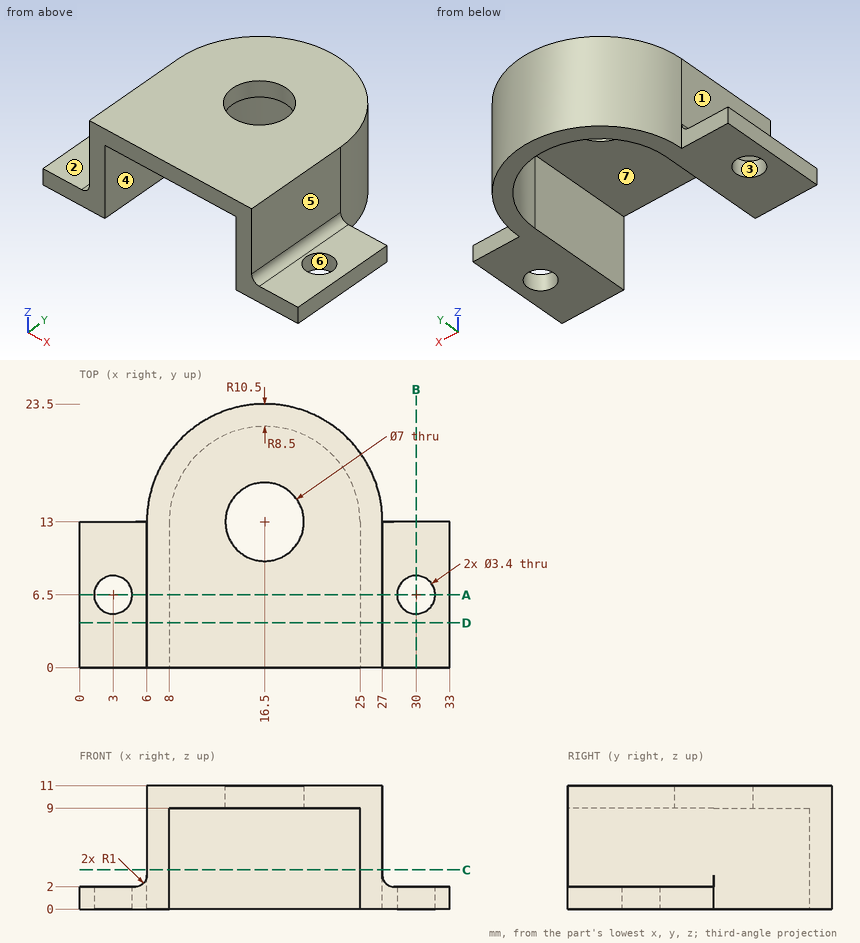
Could you check a few things on this drawing? It's one solid part, dimensions in mm from its lowest x, y, z. A direction names the side the tool comes from. Coordinates: 2 decimals unless noted, no trailing zeros. Order: outer loops, then holes, each group sorted by start corner. A loop starts at its lowest first (then second) coordinate and runs counter-clockwise, first axis right, second up.
1. If we section it at B-B (x = 30): Please give me the cut outline in (y, z).
2. For the marked faces 5, 6 and 7, which set-ups out of +Z, -Z, +X, -X, +Y, -Y let a thin tool reach every point of the face, with its end or its side?
3. If we section it at D-D (y = 4): Please give me the cut outline in (x, z), then the cut area to 3 significant figures.
4. Thinking about a two-plate mould opening in X: for the marked faces 1, 2, 3 and 4, which applies, +X half, -X half, draft (parallel to the pull), parting line (faces both ways), or undercut?
5. I'm going to push flat-ended pins straight in: pin 1 (1.5 mm diameter, centred on x = 13, y = 6.5, fed in from -Z); pin 2 (2.5 mm diameter, centred on y = 6, z = 6.5, fed in from +X); pin 3 (1.5 mm diameter, centred on x = 4, z = 1, fed in from +Y); pin 4 (4 mm diameter, centred on x = 16.5, y = 13, fed in from -Z). Where does each tip first touch, or does it pass through?
6. If we section it at A-A (y = 6.5): Please give me the cut outline in (x, z), then the cut area to 3 significant figures.
7. I need wall thicknesses on line 1 (X direction, y = 5.25, z = 6); line 2 (Y direction, x = 30, z = 0.55); line 3 (X direction, y = 13, z = 10.5). Which ranges of each line are inside material? Lowest first, please.
8. If we section it at C-C (z = 3.5): Please give me the cut outline in (x, y).
Entries:
1. outline: (0, 0) - (4.8, 0) - (4.8, 2) - (0, 2) - close; (8.2, 0) - (13, 0) - (13, 2) - (8.2, 2) - close
2. face 5: +Z, +X, +Y, -Y
2. face 6: +Z, -Z
2. face 7: -Z, -Y
3. outline: (0, 0) - (8, 0) - (8, 9) - (25, 9) - (25, 0) - (33, 0) - (33, 2) - (28, 2) arc R1 cw to (27, 3) - (27, 11) - (6, 11) - (6, 3) arc R1 cw to (5, 2) - (0, 2) - close
3. area: 102 mm2
4. face 1: -X half
4. face 2: draft
4. face 3: undercut
4. face 4: undercut
5. pin 1: stops at z = 9
5. pin 2: stops at x = 27
5. pin 3: stops at y = 13
5. pin 4: passes through
6. outline: (0, 0) - (1.3, 0) - (1.3, 2) - (0, 2) - close; (4.7, 0) - (8, 0) - (8, 9) - (25, 9) - (25, 0) - (28.3, 0) - (28.3, 2) - (28, 2) arc R1 cw to (27, 3) - (27, 11) - (6, 11) - (6, 3) arc R1 cw to (5, 2) - (4.7, 2) - close; (31.7, 0) - (33, 0) - (33, 2) - (31.7, 2) - close
6. area: 88.8 mm2
7. line 1: x = 6 to 8, 25 to 27
7. line 2: y = 0 to 4.8, 8.2 to 13
7. line 3: x = 6 to 13, 20 to 27
8. outline: (6, 0) - (8, 0) - (8, 13) arc R8.5 cw to (25, 13) - (25, 0) - (27, 0) - (27, 13) arc R10.5 ccw to (6, 13) - close
